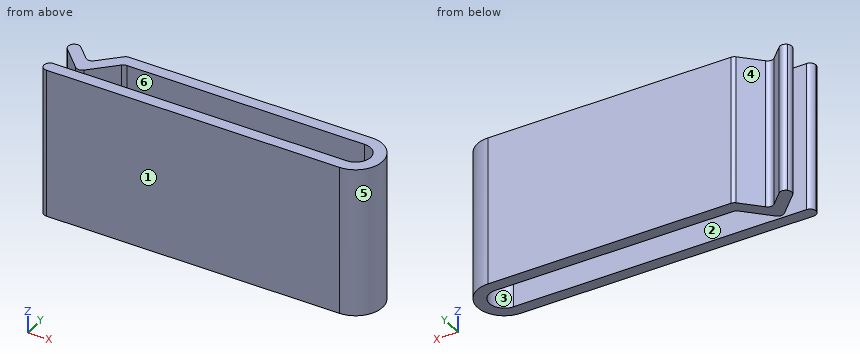
Autodesk Fusion 360 part; units mm, degrees
sketch "Sketch1" plane through (0, 0, 0) normal (0, 0, 1) x (1, 0, 0)
  line L0 (0, 0) -> (50, 0)
  arc A0 (50, 0) -> (50, 5) centre (50, 2.5) ccw
  line L1 (50, 5) -> (9.8, 5)
  line L2 (9.8, 5) -> (4.9, 0.1)
  line L3 (4.9, 0.1) -> (0, 5)
  line L4 (0, -2) -> (50, -2)
  arc A1 (50, -2) -> (50, 7) centre (50, 2.5) ccw
  line L5 (50, 7) -> (8.9716, 7)
  line L6 (8.9716, 7) -> (4.9, 2.9284)
  line L7 (4.9, 2.9284) -> (1.4142, 6.4142)
  line L8 (0, -2) -> (0, 0)
  line L9 (0, 5) -> (1.4142, 6.4142)
  dimension "d4" = 135
  dimension "d5" = 50
  dimension "d6" = 5
  dimension "d8" = 0.1
extrude "Extrude1" add sketch "Sketch1" along normal blind 25
fillet "Fillet1" radius 1 8 edges at (4.9, 2.9284, 12.5) (4.9, 0.1, 12.5) (9.8, 5, 12.5) (8.9716, 7, 12.5) (1.4142, 6.4142, 12.5) (0, 5, 12.5) (0, -2, 12.5) (0, 0, 12.5)
For this review, take the finished solid that the model builds, in its own axes (mm). Face numbers are marked on the shaded views. A direction names the side the tool comes from. Coordinates: 2 decimals unless noted, no trailing zeros. Write each loop counter-clockwise with the first axis right and the second up, starting at its lowest first coordinate (ties: lowest second). Pieces come first, ordered by that corner, then holes. Notation, with made-up numbers: (-18, 60.25) - (29, 60.25) arc R23 cw to (29, 74.25) - close; hole circle Ø10 at (-17.75, 80.5). An arc over 180 degrees is marked (long way). Answer in a Markdown table with one row per item. Add a question column.
Q1. We need section A-A, the plane x = 27.5. State the section outline as (y, z) points.
Q2. Draft analysis for pull direction Y (two halves, no side actions). For the marked faces 4, 5 and 6, state which applies: +Y half, -Y half, draft (parallel to the pull), parting line (faces both ways), or undercut.
Q3. Tool access review of the marked faces 1, 2 and 3: name each direction out of +Z, -Z, +X, -X, +Y, -Y from which nothing blocks a thin tool from reaching the whole face with its end or side.
Q4. We need section D-D, the plane y = -0.5. State the section outline as (x, z) points, and give its area (3 significant figures).
Q5. For probe 1 along Y at (x, z) = (21.5, 3.75); probe 2 along X at (y, z) = (4.25, 22.25); probe 3 along X at (y, z) = (3, 10.25), list the stretches that pass through material, from the lowest coordinate up.
Q6. We need section B-B, the plane y = 2.5. State the section outline as (x, z) points.
Q7. For P1, Ø5, axis at y = 3.5, z = 16, coming from the +X side, flat-tipped, find the tip position at first contact; note if it passes through.
Answer list:
| question | item | result |
|---|---|---|
| 1 | outline | (-2, 0) - (0, 0) - (0, 25) - (-2, 25) - close; (5, 0) - (7, 0) - (7, 25) - (5, 25) - close |
| 2 | face 4 | +Y half |
| 2 | face 5 | parting line |
| 2 | face 6 | undercut |
| 3 | face 1 | +Z, -Z, +X, -X, -Y |
| 3 | face 2 | +Z, -Z, -X |
| 3 | face 3 | +Z, -Z |
| 4 | outline | (0.13, 0) - (53.35, 0) - (53.35, 25) - (0.13, 25) - close |
| 4 | area | 1,330 mm2 |
| 5 | probe 1 | y = -2 to 0, 5 to 7 |
| 5 | probe 2 | x = 0.75 to 3.58, 6.22 to 9.05, 51.79 to 54.15 |
| 5 | probe 3 | x = 2 to 7.8, 52.45 to 54.47 |
| 6 | outline | (2.5, 0) - (7.3, 0) - (7.3, 25) - (2.5, 25) - close; (52.5, 0) - (54.5, 0) - (54.5, 25) - (52.5, 25) - close |
| 7 | P1 | stops at x = 54.5 |
